CAD build for the part. Positions are in the model's coordinates, mm. Face numbers are marked on the shaded views. A direction names the side the tool comes from. Give positions to 0.01 mm unless a question says otherwise; leave off trailing zeros. Loops run counter-clockwise (first coordinate to the right, second up) from the corner with the lowest first, then second, coordinate; pieces in that order, holes last. Notation, with made-up numbers: (25.5, -8) -> (42.5, -8) arc R13 cw to (42.5, 2) -> close; hole circle Ø1 at (33, -37.75). An arc over 180 degrees is marked (long way). Write each question's results on one line, items separated by ' | '. Start each with the question number.
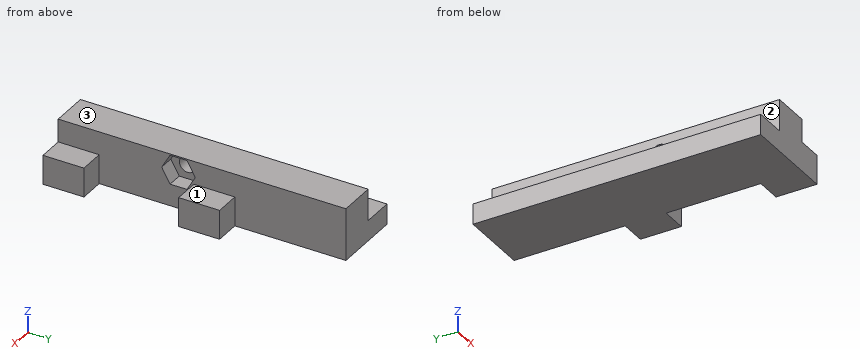
```python
from build123d import *

# Parameters (mm, degrees)
SALIENTE_EXTRUIR3_DEPTH = 4
SALIENTE_EXTRUIR4_DEPTH = 1.7
CROQUIS7_W              = 7.3
CROQUIS7_H              = 34.5
SALIENTE_EXTRUIR5_DEPTH = 4.5
CORTAR_EXTRUIR3_REACH   = 15.5
CROQUIS8_R              = 1.6
CORTAR_EXTRUIR4_DEPTH   = 3
SALIENTE_EXTRUIR6_DEPTH = 21.7


with BuildPart() as part:
    # Croquis5 → Saliente-Extruir3 (new body)
    with BuildSketch(Plane.XY):
        Polygon((18.5, 26.5), (18.5, 34.5), (0, 34.5), (0, 0), (18.5, 0), (18.5, 8), (13.5, 8), (13.5, 26.5), align=None)
    extrude(amount=SALIENTE_EXTRUIR3_DEPTH)

    # Croquis6 → Saliente-Extruir4 (add)
    with BuildSketch(Plane.XY.offset(4)):
        Polygon((6.2, 34.5), (6.2, 0), (18.5, 0), (18.5, 8), (13.5, 8), (13.5, 26.5), (18.5, 26.5), (18.5, 34.5), align=None)
    extrude(amount=SALIENTE_EXTRUIR4_DEPTH)

    # Croquis7 → Saliente-Extruir5 (add)
    with BuildSketch(Plane.XY.offset(5.7)):
        with Locations((9.85, 17.25)):
            Rectangle(CROQUIS7_W, CROQUIS7_H)
    extrude(amount=SALIENTE_EXTRUIR5_DEPTH)

    # Croquis8 → Cortar-Extruir3 (cut, up to next)
    with BuildSketch(Plane(origin=(13.5, 0, 0), x_dir=(0, 0, -1), z_dir=(1, 0, 0)), mode=Mode.PRIVATE) as cortar_extruir3_sk1:
        with Locations((-7.1, 23.5)):
            Circle(CROQUIS8_R)
    cortar_extruir3_tool1 = extrude(cortar_extruir3_sk1.sketch, amount=-CORTAR_EXTRUIR3_REACH, mode=Mode.PRIVATE) & part.part
    add(cortar_extruir3_tool1.solids().sort_by_distance((13.5, 23.5, 7.1))[0], mode=Mode.SUBTRACT)

    # Croquis9 → Cortar-Extruir4 (cut)
    with BuildSketch(Plane(origin=(13.5, 0, 0), x_dir=(0, 0, -1), z_dir=(1, 0, 0))):
        Polygon((-7.1, 26.790896534), (-9.95, 25.145448267), (-9.95, 21.854551733), (-7.1, 20.209103466), (-4.25, 21.854551733), (-4.25, 25.145448267), align=None)
    extrude(amount=-CORTAR_EXTRUIR4_DEPTH, mode=Mode.SUBTRACT)

    # Croquis10 → Saliente-Extruir6 (add)
    with BuildSketch(Plane(origin=(0, 34.5, 0), x_dir=(1, 0, 0), z_dir=(0, 1, 0))):
        Polygon((13.5, -5.7), (13.5, 0), (0, 0), (0, -4), (6.2, -4), (6.2, -10.2), (13.5, -10.2), align=None)
    extrude(amount=SALIENTE_EXTRUIR6_DEPTH)


solid = part.part
```
Q1. Saw through at C-C, the plane z = 3. List the corners of the cut face in (x, y).
Q2. Saw through at D-D, the plane z = 6.5. List the corners of the cut face in (x, y), then the cut area to 3 significant figures.
Q3. Saw through at A-A, the plane y = 31. List the corners of the cut face in (x, z), then the cut area to 3 significant figures.
Q4. Which spindle directions (+Z, -Z, +X, -X, +Y, -Y) get a long thin tool onto all of the face, cutting with end or side? Do the marked faces 1, 2 and 3. Say none if no direction does.
Q5. Wall check: L1, parallel to Y at x = 7.55, z = 7.1; L2, parallel to X at y = 32, z = 9.25; L3, parallel to X at y = 4, z = 4.5. Give the ranges that are in metal, low to high.
Q6. Drop flat-ended pins along their axis: pin 1 (5 mm diameter, centred on y = 31, z = 8.5, fed in from -X); pin 2 (2.5 mm diameter, centred on x = 17, z = 4, fed in from +Y); pin 3 (2.5 mm diameter, centred on x = 15.5, y = 28.5, fed in from +Z). Give the stop position or say it passes through.
Q7. Saw through at B-B, the plane y = 23.5. List the corners of the cut face in (x, z), then the cut area to 3 significant figures.
Answer block:
1) outline: (0, 0) -> (18.5, 0) -> (18.5, 8) -> (13.5, 8) -> (13.5, 26.5) -> (18.5, 26.5) -> (18.5, 34.5) -> (13.5, 34.5) -> (13.5, 56.2) -> (0, 56.2) -> close
2) outline: (6.2, 0) -> (13.5, 0) -> (13.5, 20.56) -> (10.5, 20.56) -> (10.5, 22.02) -> (6.2, 22.02) -> close; (6.2, 24.98) -> (10.5, 24.98) -> (10.5, 26.44) -> (13.5, 26.44) -> (13.5, 56.2) -> (6.2, 56.2) -> close | area: 380 mm2
3) outline: (0, 0) -> (18.5, 0) -> (18.5, 5.7) -> (13.5, 5.7) -> (13.5, 10.2) -> (6.2, 10.2) -> (6.2, 4) -> (0, 4) -> close | area: 128 mm2
4) face 1: +Z, +X, +Y, -Y | face 2: +Z, -X, +Y, -Y | face 3: +Z, +X, -X, +Y, -Y
5) L1: y = 0 to 21.9, 25.1 to 56.2 | L2: x = 6.2 to 13.5 | L3: x = 6.2 to 18.5
6) pin 1: stops at x = 6.2 | pin 2: stops at y = 34.5 | pin 3: stops at z = 5.7
7) outline: (0, 0) -> (13.5, 0) -> (13.5, 4.25) -> (10.5, 4.25) -> (10.5, 5.5) -> (6.2, 5.5) -> (6.2, 4) -> (0, 4) -> close; (6.2, 8.7) -> (10.5, 8.7) -> (10.5, 9.95) -> (13.5, 9.95) -> (13.5, 10.2) -> (6.2, 10.2) -> close | area: 68.4 mm2
